For this review, use the dimensioned drawing (mm, ordinates from the lowest corner) and the shaded views. A direction names the side the tool comes from. Coordinates: 2 decimals unless noted, no trailing zeros. Loops run counter-clockwise (first coordinate to the right, second up) from the corner with the lowest first, then second, coordinate; pieces in that order, holes last. Notation, with made-up numbers: (82.5, -15) - (113.5, -15) arc R22 cw to (113.5, 15) - close; hole circle Ø11 at (-20.75, 4.25). An arc over 180 degrees is marked (long way). Use one line per item in the form item = value. Start each with the question number.
(1) Add section A-A (x = 11). State the section outline as (y, z) points, plus the area to 3 significant figures.
(2) Add section B-B (y = 10). State the section outline as (x, z) points.
(3) Add section D-D (y = 8.1). State the section outline as (x, z) points.
(4) The part is to be moulded in two halves that separate along Y. For the marked faces 1, 2 and 3, say which applies: pulls with the +Y half, pulls with the -Y half, needs draft (parallel to the pull), parting line crosses it, or undercut.
(5) Tool access review of the marked faces 4, 5 and 6: name each direction out of +Z, -Z, +X, -X, +Y, -Y from which nothing blocks a thin tool from reaching the whole face with its end or side.
(6) Add section C-C (z = 1.9). State the section outline as (x, y) points.
(7) Clearance check with flat-ended pins moving along their axes: pin 1 Ø1.5 at (x, z) = (31.5, 2) entering from +Y; pin 2 Ø1.2 at (y, z) = (6, 2.5) entering from -X. State where each tip first meets the part, or that it passes through.
(8) For L1, parallel to X at y = 3.5, z = 2.4; L2, parallel to Y at x = 24, z = 0.9; L3, parallel to X at y = 8, z = 3.05, list the stretches that pass through material, from the lowest coordinate up.
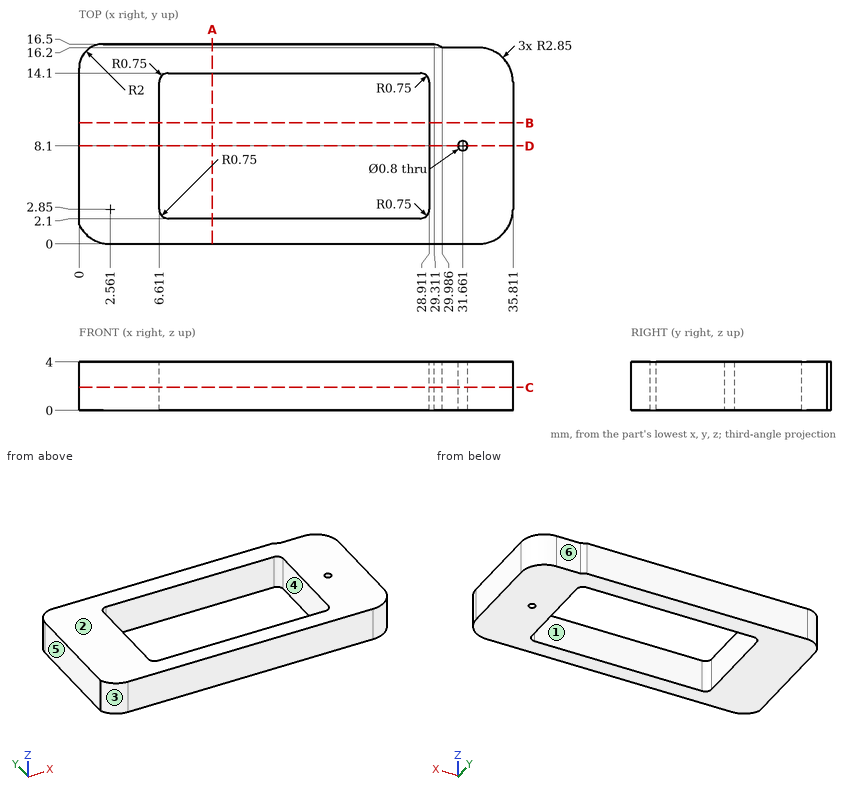
Computed values:
q1.outline = (0, 0) - (2.1, 0) - (2.1, 4) - (0, 4) - close; (14.1, 0) - (16.5, 0) - (16.5, 4) - (14.1, 4) - close
q1.area = 18.0 mm^2
q2.outline = (0, 0) - (6.61, 0) - (6.61, 4) - (0, 4) - close; (28.91, 0) - (35.81, 0) - (35.81, 4) - (28.91, 4) - close
q3.outline = (0, 0) - (6.61, 0) - (6.61, 4) - (0, 4) - close; (28.91, 0) - (31.26, 0) - (31.26, 4) - (28.91, 4) - close; (32.06, 0) - (35.81, 0) - (35.81, 4) - (32.06, 4) - close
q4.face_1 = undercut
q4.face_2 = needs draft
q4.face_3 = pulls with the -Y half
q5.face_4 = +Z, -Z
q5.face_5 = +Z, -Z, -X, +Y, -Y
q5.face_6 = +Z, -Z, +X, +Y
q6.outline = (0, 1.6) arc R2.85 ccw to (2.56, 0) - (32.96, 0) arc R2.85 ccw to (35.81, 2.85) - (35.81, 13.35) arc R2.85 ccw to (32.96, 16.2) - (29.99, 16.2) - (29.31, 16.5) - (2, 16.5) arc R2 ccw to (0, 14.5) - close; hole (6.61, 2.85) arc R0.75 ccw to (7.36, 2.1) - (28.16, 2.1) arc R0.75 ccw to (28.91, 2.85) - (28.91, 13.35) arc R0.75 ccw to (28.16, 14.1) - (7.36, 14.1) arc R0.75 ccw to (6.61, 13.35) - close; hole circle Ø0.8 at (31.66, 8.1)
q7.pin_1 = 16.2
q7.pin_2 = 0
q8.L1 = 0 to 6.61, 28.91 to 35.81
q8.L2 = 0 to 2.1, 14.1 to 16.5
q8.L3 = 0 to 6.61, 28.91 to 31.27, 32.05 to 35.81
